Geometry: final body of the model. Coordinates: model frame, mm. A direction names the side the tool comes from. Give positions to 0.01 mm unless a question says otherwise; leave off trailing zeros. Write each loop counter-clockwise with the first axis right and the second up, starting at its lowest first coordinate (ties: lowest second). Pieces come first, ordered by that corner, then holes. Notation, with made-up numbers: (69.5, 44) -> (103.5, 44) arc R21 cw to (103.5, 66) -> close; hole circle Ø2 at (-23, 55). An arc over 180 degrees is marked (long way). Answer as a JSON object with one key per item and string values. Group by question number.
(1) Material intervals for probe 1 along Y at (x, z) = (25, 47.5); probe 2 along X at (y, z) = (-8, -1.5) (3 decimals); probe 3 along Z at (x, y) = (23, -47.5) (3 decimals), sorted ascending.
(2) Set-up query: faces 1 (the face through (60.325, 0, 52)), 2 (the face through (59, 0, 42.875)), 3 (the face through (1, -45, 9.525)), 4 (the face through (10, 25.4, 30)), 5 (the face through (-41.275, -1, 0)). Return all of +Z, -Z, +X, -X, +Y, -Y with unobstructed straight access to the full face (end or side cutting, diameter ignored); none if empty.
(3) Contact query for flat-ended pins moving along their axis: pin 1 Ø2 at (y, z) = (-27.5, 53.5) entering from -X; pin 2 Ø11.5 at (x, y) = (-7, -42.5) entering from +Z (3 decimals); pin 3 Ø12 at (x, y) = (-22.5, -23) entering from +Z; pin 4 Ø1.5 at (x, z) = (6, 38.5) entering from -Y. Output: stop coordinate, or through.
(4) Section query A-A on z = -3. Output: boundary loops of the cut face in (x, y) (3 decimals), plus the area to 3 significant figures.
(5) Section query B-B on y = -30.5. Output: boundary loops of the cut face in (x, z) (3 decimals).
from build123d import *

# Parameters (mm, degrees)
F1_DEPTH = 63.5
F2_DEPTH = 25.4


with BuildPart() as f1:
    # F0 (on Front) → F1 (new body, symmetric)
    with BuildSketch(Plane.XZ):
        Polygon((-41.275, -9.525), (41.275, -9.525), (41.275, 9.525), (22.225, 9.525), (-41.275, 9.525), align=None)
    extrude(amount=F1_DEPTH, both=True)

    # F0 (on Front) → F2 (join, symmetric)
    with BuildSketch(Plane.XZ):
        with BuildLine():
            add(Edge.make_bspline(
                [(-41.275, 9.525), (-40.101912, 24.682952), (16.535287, 61.9252), (57.15, 61.9252)],
                knots=[0, 0, 0, 0, 111.504536, 111.504536, 111.504536, 111.504536], degree=3))
            Line((-41.275, 9.525), (22.225, 9.525))
            Line((22.225, 9.525), (22.225, 27.0002))
            ThreePointArc((22.225, 27.0002), (32.454296, 51.695904), (57.15, 61.9252))
        make_face()
        with BuildLine():
            Line((22.225, 9.525), (41.275, 9.525))
            Line((41.275, 9.525), (41.275, 27.0002))
            ThreePointArc((41.275, 27.0002), (45.92468, 38.22552), (57.15, 42.8752))
            Line((57.15, 42.8752), (60.325, 42.8752))
            Line((60.325, 42.8752), (60.325, 61.9252))
            Line((60.325, 61.9252), (57.15, 61.9252))
            ThreePointArc((57.15, 61.9252), (32.454296, 51.695904), (22.225, 27.0002))
            Line((22.225, 27.0002), (22.225, 9.525))
        make_face()
    extrude(amount=F2_DEPTH, both=True)


solid = f1.part
Answer list:
{
 "1": {"probe 1": "-25.4 to 25.4", "probe 2": "-41.275 to 41.275", "probe 3": "-9.525 to 9.525"},
 "2": {"face 1": "+Z, -Z, +X, +Y, -Y", "face 2": "-Z, +X, +Y, -Y", "face 3": "+Z, +X, -X, -Y", "face 4": "+Z, +X, -X, +Y", "face 5": "+Z, -Z, -X, +Y, -Y"},
 "3": {"pin 1": "through", "pin 2": "z = 9.525", "pin 3": "z = 35.41", "pin 4": "y = -25.4"},
 "4": {"outline": "(-41.275, -63.5) -> (41.275, -63.5) -> (41.275, 63.5) -> (-41.275, 63.5) -> close", "area": "10,500 mm2"},
 "5": {"outline": "(-41.275, -9.525) -> (41.275, -9.525) -> (41.275, 9.525) -> (-41.275, 9.525) -> close"}
}
